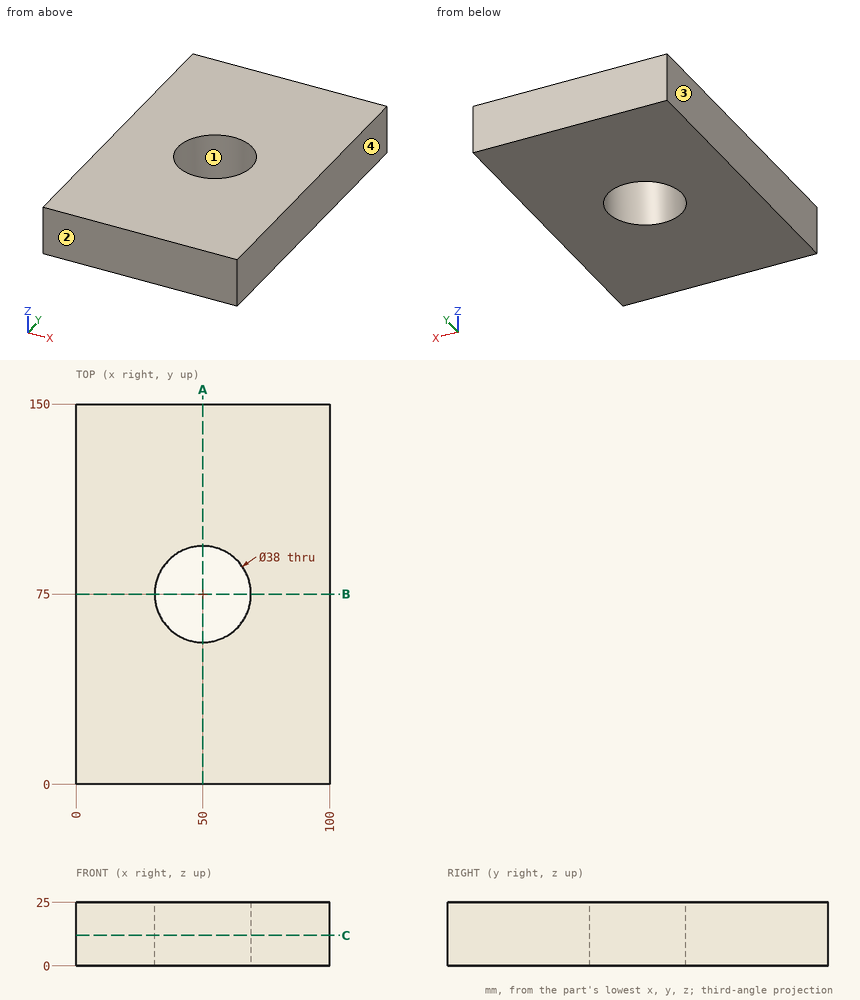
For this review, use the dimensioned drawing (mm, ordinates from the lowest corner) and the shaded views. Coordinates: 2 decimals unless noted, no trailing zeros. Order: outer loops, then holes, each group sorted by start corner. A loop starts at its lowest first (then second) coordinate and runs counter-clockwise, first axis right, second up. Notation, with made-up numbers: (53, -21) - (92, -21) arc R21 ccw to (92, 0) - close; hole circle Ø7 at (15, 81.25). An arc over 180 degrees is marked (long way). Answer as a JSON object with one key per item and string values. Group by question number.
1. We need section B-B on y = 75. State the section outline as (x, z) points, then the cut area to 3 significant figures.
2. We need section C-C on z = 12. State the section outline as (x, y) points.
3. Clearance check with a flat-ended pin moving along its axis: P1, Ø5, axis at x = 50, y = 89, coming from the +Z side. State where the tip first meets the part, or that it passes through.
4. The part is to be moulded in two halves that separate along X. For the marked faces 1, 2, 3 and 4, say which applies: pulls with the +X half, pulls with the -X half, needs draft (parallel to the pull), parting line crosses it, or undercut.
5. For probe 1 along Y at (x, z) = (50, 9.25); probe 2 along X at (y, z) = (63, 18.5); probe 3 along X at (y, z) = (84, 6), list the stretches that pass through material, from the lowest coordinate up.
6. We need section A-A on x = 50. State the section outline as (y, z) points, then the cut area to 3 significant figures.
Final values:
{
 "1": {"outline": "(0, 0) - (31, 0) - (31, 25) - (0, 25) - close; (69, 0) - (100, 0) - (100, 25) - (69, 25) - close", "area": "1,550 mm²"},
 "2": {"outline": "(0, 0) - (100, 0) - (100, 150) - (0, 150) - close; hole circle Ø38 at (50, 75)"},
 "3": {"P1": "through"},
 "4": {"face 1": "undercut", "face 2": "needs draft", "face 3": "pulls with the -X half", "face 4": "pulls with the +X half"},
 "5": {"probe 1": "0 to 56, 94 to 150", "probe 2": "0 to 35.27, 64.73 to 100", "probe 3": "0 to 33.27, 66.73 to 100"},
 "6": {"outline": "(0, 0) - (56, 0) - (56, 25) - (0, 25) - close; (94, 0) - (150, 0) - (150, 25) - (94, 25) - close", "area": "2,800 mm²"}
}
